```python
from build123d import *

# Parameters (mm, degrees)
F0_W     = 50
F0_H     = 50.8
F1_DEPTH = 750
F2_R     = 5
F3_T     = -2.5


with BuildPart() as f1:
    # F0 (on Top) → F1 (new body)
    with BuildSketch(Plane.XY):
        with Locations((0, -0.4)):
            Rectangle(F0_W, F0_H)
    extrude(amount=F1_DEPTH)

    # F2
    f2_edges = [f1.edges().sort_by_distance(p)[0] for p in [
        (25, 25, 375),
        (25, -25.8, 375),
        (-25, 25, 375),
        (-25, -25.8, 375),
    ]]
    fillet(f2_edges, radius=F2_R)

    # F3
    f3_openings = [f1.faces().sort_by_distance(p)[0] for p in [
        (0, -0.4, 750),
        (0, -0.4, 0),
    ]]
    offset(amount=F3_T, openings=f3_openings)


solid = f1.part
```
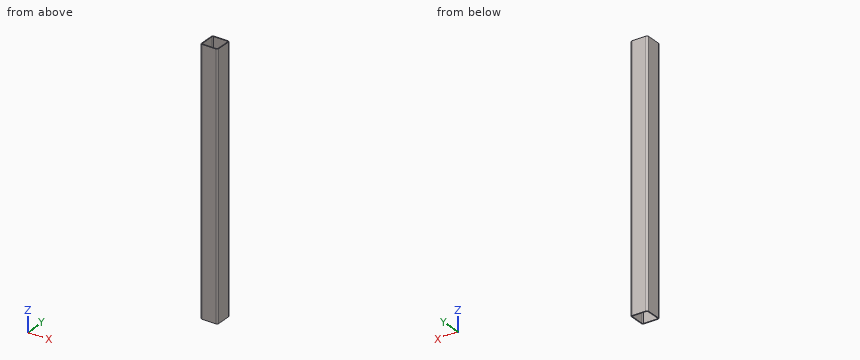
The model under review builds one solid part; all positions refer to its coordinate system, in mm. Give positions to 0.01 mm unless a question says otherwise; leave off trailing zeros. Write each loop counter-clockwise with the first axis right and the second up, starting at its lowest first coordinate (ties: lowest second). Pieces come first, ordered by that corner, then holes. Notation, with made-up numbers: M 52.25,55.5 L 93.25,55.5 A16 ccw 93.25,73.5 Z; hole C 23,58.25 d9. An arc over 180 degrees is marked long. Write each question's results on one line, items separated by ' | '. Start each with the question number.
1. We need section B-B (y = -2). Write out the cut boundary in (x, z).
2. We need section C-C (x = 4). Write out the cut boundary in (y, z), and give its area (3 significant figures).
3. For probe 1 along X at (y, z) = (-13, 630); probe 2 along Y at (x, z) = (10, 310); probe 3 along Y at (x, z) = (21.5, 79.5), list the stretches that pass through material, from the lowest coordinate up. Write a range as [from, to].
4. We need section A-A (z = 648.5). Write out the cut boundary in (x, y).
Results found:
1) outline: M -25,0 L -22.5,0 L -22.5,750 L -25,750 Z; M 22.5,0 L 25,0 L 25,750 L 22.5,750 Z
2) outline: M -25.8,0 L -23.3,0 L -23.3,750 L -25.8,750 Z; M 22.5,0 L 25,0 L 25,750 L 22.5,750 Z | area: 3,750 mm^2
3) probe 1: x = [-25, -22.5], [22.5, 25] | probe 2: y = [-25.8, -23.3], [22.5, 25] | probe 3: y = [-25.57, -22.8], [22, 24.77]
4) outline: M -25,-20.8 A5 ccw -20,-25.8 L 20,-25.8 A5 ccw 25,-20.8 L 25,20 A5 ccw 20,25 L -20,25 A5 ccw -25,20 Z; hole M -22.5,-20.8 A2.5 ccw -20,-23.3 L 20,-23.3 A2.5 ccw 22.5,-20.8 L 22.5,20 A2.5 ccw 20,22.5 L -20,22.5 A2.5 ccw -22.5,20 Z
